Design review of the part shown in the three views and the two pictorial views. Dimensions are in mm from the part's minimum x, y and z. Coordinates: 2 decimals unless noted, no trailing zeros. Write each loop counter-clockwise with the first axis right and the second up, starting at its lowest first coordinate (ties: lowest second). Pieces come first, ordered by that corner, then holes. Notation, with made-up numbers: (9.25, 22.5) - (39.25, 22.5) arc R26 cw to (39.25, 61.5) - close; hole circle Ø8 at (15, 37). An arc over 180 degrees is marked (long way). Return JSON: item names as keys, results as strings. Group by question number.
(1) We need section C-C on x = 21. State the section outline as (y, z) points, then the cut area to 3 significant figures.
(2) We need section B-B on x = 35. State the section outline as (y, z) points (1 decimal).
(3) For pin 1 Ø1.5 at (x, y) = (58, 2.5) entering from +Z; pin 2 Ø1.5 at (y, z) = (2.5, 85) entering from -X, all flat-tipped, find the tip position at first contact; note any pin that passes through.
(4) To check wall thickness, follow L1, parallel to Z at x = 35, y = 2.75 (1 decimal); L2, parallel to Z at x = 6.5, y = 2.75; L3, parallel to X at y = 4.8, z = 85.5. State the ranges of each line that lie inside material, in increasing order. Write a range as from..to.
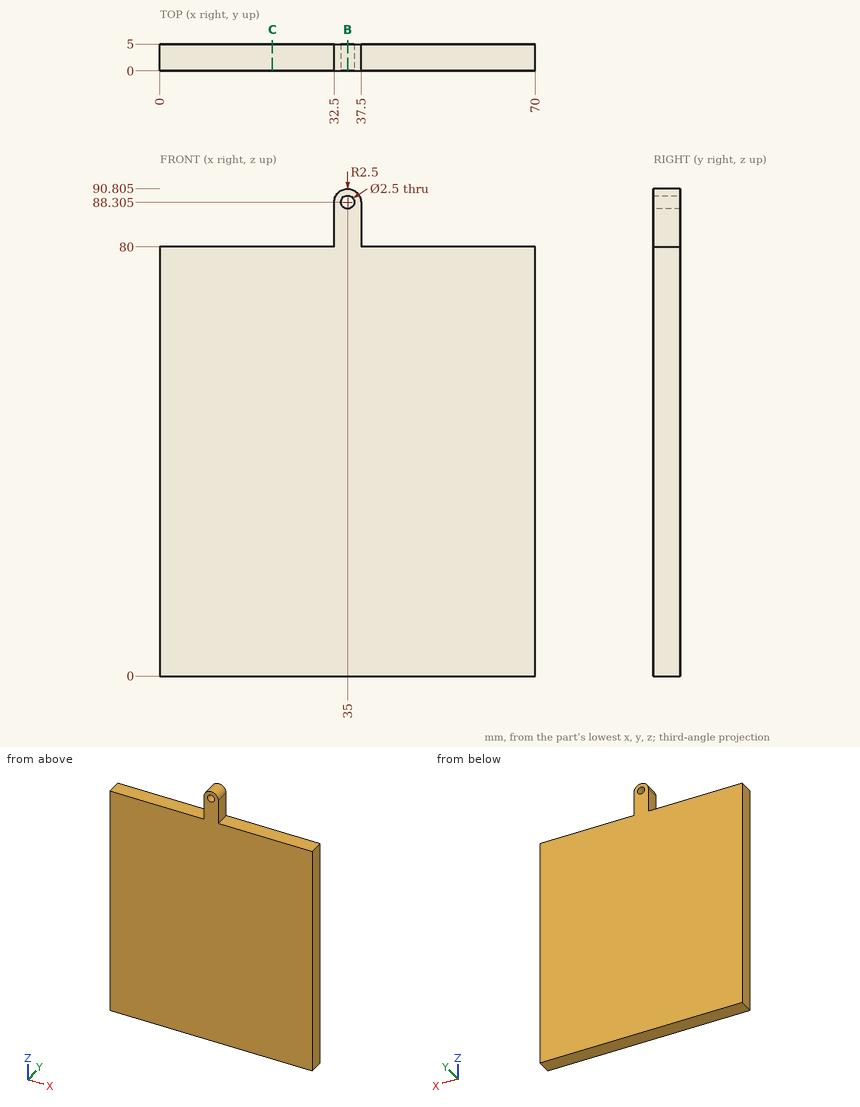
Ans:
{
 "1": {"outline": "(0, 0) - (5, 0) - (5, 80) - (0, 80) - close", "area": "400 mm²"},
 "2": {"outline": "(0, 0) - (5, 0) - (5, 87.1) - (0, 87.1) - close; (0, 89.6) - (5, 89.6) - (5, 90.8) - (0, 90.8) - close"},
 "3": {"pin 1": "z = 80", "pin 2": "x = 32.5"},
 "4": {"L1": "0..87.1, 89.6..90.8", "L2": "0..80", "L3": "32.5..37.5"}
}
